The drawing under review shows one solid part. Ordinate dimensions are in mm from its lowest x, y, z. Round coordinates to 2 decimals unless told otherwise and drop trailing zeros. Write each loop counter-clockwise with the first axis right and the second up, starting at its lowest first coordinate (ties: lowest second). Pieces come first, ordered by that corner, then holes. Notation, with made-up numbers: (3.25, -19) -> (22.25, -19) arc R18 ccw to (22.25, 1) -> close; hole circle Ø3 at (-14, 51.25). An arc over 180 degrees is marked (long way). Write item = value, one per line. Start each with the question number.
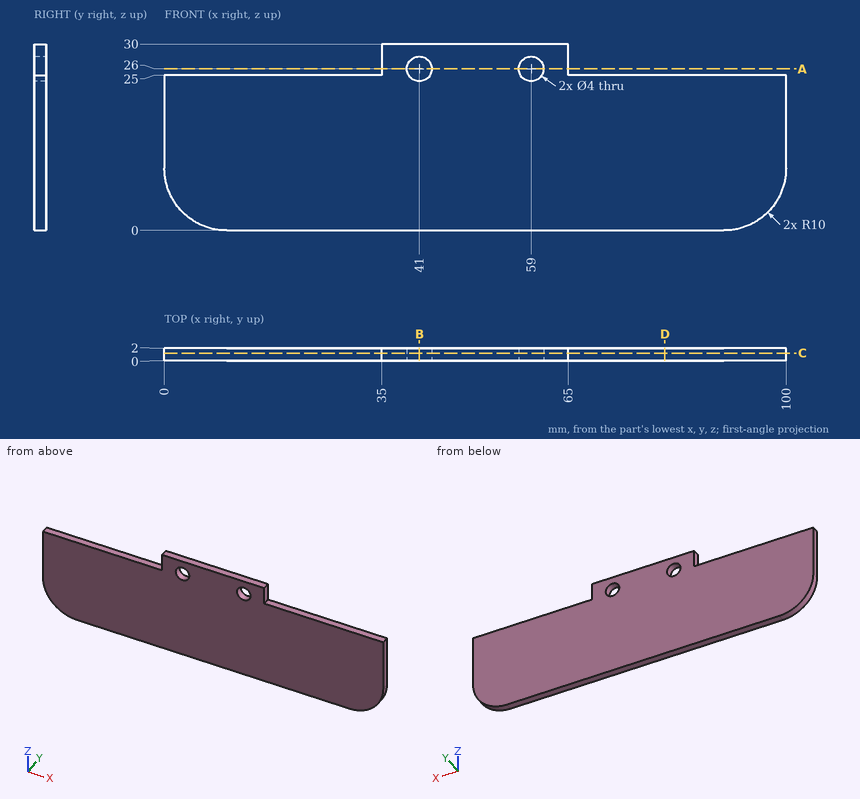
1. Clearance check with flat-ended pins moving along their axes: pin 1 Ø2.5 at (x, z) = (59, 26) entering from -Y; pin 2 Ø1 at (x, y) = (75.5, 1.5) entering from +Z. State where each tip first meets the part, or that it passes through.
2. Consider section A-A, the plane z = 26. Give the boundary of the cut face in (x, y), then the cut area to 3 significant figures.
3. Consider section D-D, the plane x = 80.5. Give the boundary of the cut face in (y, z), then the cut area to 3 significant figures.
4. Consider section B-B, the plane x = 41. Give the boundary of the cut face in (y, z), then the cut area to 3 significant figures.
5. Wall thickness on L1, parallel to X at y = 0.4, z = 26; L2, parallel to Z at x = 71.5, y = 0.1; L3, parallel to X at y = 0.2, z = 5: over which ranges is each line inside the solid? List them lowest first. Write a range as from..to.
6. Consider section C-C, the plane y = 1.25. Give the boundary of the cut face in (x, z).
Outcome:
q1.pin_1 = through
q1.pin_2 = 25
q2.outline = (35, 0) -> (39, 0) -> (39, 2) -> (35, 2) -> close; (43, 0) -> (57, 0) -> (57, 2) -> (43, 2) -> close; (61, 0) -> (65, 0) -> (65, 2) -> (61, 2) -> close
q2.area = 44.0 mm2
q3.outline = (0, 0) -> (2, 0) -> (2, 25) -> (0, 25) -> close
q3.area = 50.0 mm2
q4.outline = (0, 0) -> (2, 0) -> (2, 24) -> (0, 24) -> close; (0, 28) -> (2, 28) -> (2, 30) -> (0, 30) -> close
q4.area = 52.0 mm2
q5.L1 = 35..39, 43..57, 61..65
q5.L2 = 0..25
q5.L3 = 1.34..98.66
q6.outline = (0, 10) arc R10 ccw to (10, 0) -> (90, 0) arc R10 ccw to (100, 10) -> (100, 25) -> (65, 25) -> (65, 30) -> (35, 30) -> (35, 25) -> (0, 25) -> close; hole circle Ø4 at (41, 26); hole circle Ø4 at (59, 26)
